Work out the finished part from the listing and answer in its coordinate system (mm). Face numbers are marked on the shaded views. A direction names the side the tool comes from. Round coordinates to 2 decimals unless told otherwise and drop trailing zeros. Loops run counter-clockwise (first coordinate to the right, second up) from the corner with the lowest first, then second, coordinate; pieces in that order, holes last. Notation, with made-up numbers: (-5.75, 74.25) - (-0.75, 74.25) arc R15 ccw to (-0.75, 103.25) - close; hole circle Ø6 at (-27, 67.5). An arc over 180 degrees is marked (long way). Answer as CSV lines item,"result". Start each with the question number.
```python
from build123d import *

# Parameters (mm, degrees)
SKETCH1_R           = 227.5
BOSS_EXTRUDE1_DEPTH = 7.5
BOSS_EXTRUDE2_START = 7.5
SKETCH1_3_R         = 15
BOSS_EXTRUDE2_DEPTH = 35
SKETCH2_R           = 40
SKETCH2_R_2         = 30
CUT_EXTRUDE1_DEPTH  = 16
BOSS_EXTRUDE3_START = -7.5
SKETCH3_R           = 15
BOSS_EXTRUDE3_DEPTH = 74.827954589


with BuildPart() as part:
    # Sketch1 → Boss-Extrude1 (new body, symmetric)
    with BuildSketch(Plane.XY):
        Circle(SKETCH1_R)
    extrude(amount=BOSS_EXTRUDE1_DEPTH, both=True)

    # Sketch1<3> → Boss-Extrude2 (add)
    with BuildSketch(Plane.XY.offset(BOSS_EXTRUDE2_START)):
        with Locations((0, 200)):
            Circle(SKETCH1_3_R)
    extrude(amount=BOSS_EXTRUDE2_DEPTH)

    # Sketch2 → Cut-Extrude1 (cut, through all)
    with BuildSketch(Plane.XY.offset(7.5)):
        with Locations((-172.341356777, 30.388431092)):
            Circle(SKETCH2_R)
        with Locations((0, 100)):
            Circle(SKETCH2_R_2)
        with Locations((90.630778704, 42.261826174)):
            Circle(SKETCH2_R_2)
        with Locations((-90.630778704, -42.261826174)):
            Circle(SKETCH2_R_2)
        with Locations((112.487831695, 134.057777546)):
            Circle(SKETCH2_R)
        with Locations((59.853525082, -164.446208638)):
            Circle(SKETCH2_R)
    extrude(amount=-CUT_EXTRUDE1_DEPTH, mode=Mode.SUBTRACT)

    # Sketch3 → Boss-Extrude3 (add)
    with BuildSketch(Plane.XY.offset(BOSS_EXTRUDE3_START)):
        Circle(SKETCH3_R)
    extrude(amount=-BOSS_EXTRUDE3_DEPTH)


solid = part.part
```
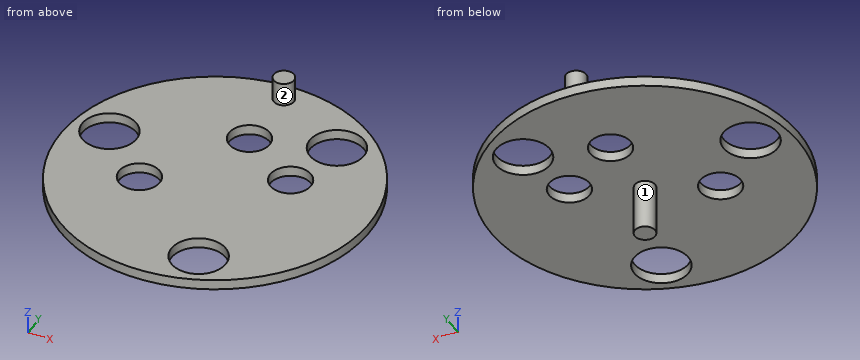
Item 1: Section D-D, the plane x = -72 is taken. Give the vertices of the cut face in (y, z), and give its area (3 significant figures).
Item 2: Find the intervals of material crossed by L1, parallel to Y at x = 0, z = 2.75; L2, parallel to Z at x = -133, y = 94; L3, parallel to X at y = 94, z = 4.5, in increasing order.
Item 3: Flat-ended cylindrical pins translate along their axes: pin 1 Ø12 at (x, y) = (-111, 28) entering from -Z; pin 2 Ø4 at (y, z) = (101.5, -8.5) entering from -X. Find the tip coordinate at first contact, or state that the pin passes through.
Item 4: Which of the six approach directions +Z, -Z, +X, -X, +Y, -Y give full straight-line access (tool end or side, diameter ignored) to the marked faces 1 and 2?
Item 5: Section A-A, the plane x = 0 is taken. Give the vertices of the cut face in (y, z).
Item 6: Section B-B, the plane y = 0 is taken. Give the vertices of the cut face in (x, z), and give its area (3 significant figures).
Item 7: Section C-C, the plane y = 200 is taken. Give the vertices of the cut face in (x, z).
Answer:
1,outline,"(-215.81, -7.5) - (-65.78, -7.5) - (-65.78, 7.5) - (-215.81, 7.5) - close; (-18.75, -7.5) - (215.81, -7.5) - (215.81, 7.5) - (-18.75, 7.5) - close"
1,area,"5,770 mm²"
2,L1,"y = -227.5 to 70, 130 to 227.5"
2,L2,"z = -7.5 to 7.5"
2,L3,"x = -207.17 to -29.39, 29.39 to 207.17"
3,pin 1,"stops at z = -7.5"
3,pin 2,"stops at x = -204.46"
4,face 1,"-Z"
4,face 2,"+Z"
5,outline,"(-227.5, -7.5) - (-15, -7.5) - (-15, -82.33) - (15, -82.33) - (15, -7.5) - (70, -7.5) - (70, 7.5) - (-227.5, 7.5) - close; (130, -7.5) - (227.5, -7.5) - (227.5, 7.5) - (215, 7.5) - (215, 42.5) - (185, 42.5) - (185, 7.5) - (130, 7.5) - close"
6,outline,"(-227.5, -7.5) - (-198.35, -7.5) - (-198.35, 7.5) - (-227.5, 7.5) - close; (-146.33, -7.5) - (-15, -7.5) - (-15, -82.33) - (15, -82.33) - (15, -7.5) - (227.5, -7.5) - (227.5, 7.5) - (-146.33, 7.5) - close"
6,area,"8,290 mm²"
7,outline,"(-108.43, -7.5) - (108.43, -7.5) - (108.43, 7.5) - (15, 7.5) - (15, 42.5) - (-15, 42.5) - (-15, 7.5) - (-108.43, 7.5) - close"
